Here's how the part is built. I have some questions about the finished solid (model axes, mm). Face numbers are marked on the shaded views. A direction names the side the tool comes from. Coordinates: 2 decimals unless noted, no trailing zeros. Loops run counter-clockwise (first coordinate to the right, second up) from the corner with the lowest first, then second, coordinate; pieces in that order, holes last.
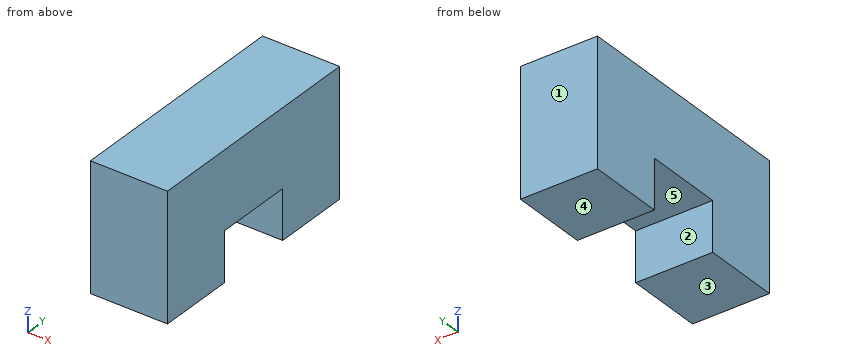
Autodesk Inventor part; units mm, degrees
ref_plane "YZ Plane" through (0, 0, 0) normal (1, 0, 0) x (0, 1, 0)
ref_plane "XZ Plane" through (0, 0, 0) normal (0, 1, 0) x (-1, 0, 0)
ref_plane "XY Plane" through (0, 0, 0) normal (0, 0, 1) x (1, 0, 0)
sketch "Sketch1" plane through (0, 0, 0) normal (0, 0, 1) x (1, 0, 0)
  line L0 (0, 0) -> (39, 0)
  line L1 (39, 0) -> (39, 39)
  line L2 (39, 39) -> (0, 39)
  line L3 (0, 39) -> (0, 0)
  dimension "d0" = 39
  dimension "d1" = 39
sketch "Sketch2" plane through (0, 0, 0) normal (1, 0, 0) x (0, 1, 0)
  line L0 (0, 0) -> (0, 25)
  line L1 (0, 25) -> (-40, 25)
  line L2 (-40, 25) -> (-40, 0)
  dimension "d2" = 25
  dimension "d3" = 40
sweep "Sweep1" add profiles "Sketch1" path "Sketch2"
properties part number "motor support"
Q1. Please list where these lines run through material, in increasing order: probe 1 along Y at (x, z) = (16, 11.5); probe 2 along Z at (x, y) = (18, -22).
Q2. Suppose I cut it at C-C on y = -28. Write out the boundary of the cut face in (x, z).
Q3. Suppose I cut it at A-A on z = 6. Write out the boundary of the cut face in (x, y).
Q4. Will this pin go through, and if not, where does the flat tip stop? P1, Ø19.5, axis at x = 18, y = -12.5, coming from the -Z side.
Q5. For the marked faces 4 and 5, which set-ups out of +Z, -Z, +X, -X, +Y, -Y let a thin tool reach every point of the face, with its end or its side?
Q6. We'd pull the mould along Y, two halves only. Please class the marked faces 1, 2 and 3: pulls with the +Y half, pulls with the -Y half, needs draft (parallel to the pull), parting line crosses it, or undercut.
Q7. Suppose I cut it at B-B on x = 28.5. Write out the boundary of the cut face in (y, z).
Check values:
1. probe 1: y = -79 to -40, 0 to 39
1. probe 2: z = 25 to 64
2. outline: (0, 25) - (39, 25) - (39, 64) - (0, 64) - close
3. outline: (0, -79) - (39, -79) - (39, -40) - (0, -40) - close; (0, 0) - (39, 0) - (39, 39) - (0, 39) - close
4. P1: stops at z = 25
5. face 4: -Z, +X, -X, +Y, -Y
5. face 5: -Z, +X, -X
6. face 1: pulls with the +Y half
6. face 2: undercut
6. face 3: needs draft
7. outline: (-79, 0) - (-40, 0) - (-40, 25) - (0, 25) - (0, 0) - (39, 0) - (39, 64) - (-79, 64) - close
